from build123d import *

# Parameters (mm, degrees)
SM_BASE_FLANGE_1_DEPTH = 40
SKETCH_6_R             = 1.7
CUT_EXTRUDE_1_DEPTH    = 10
SKETCH_7_R             = 1.7
CUT_EXTRUDE_2_DEPTH    = 10
SKETCH_11_W            = 25.332346726
SKETCH_11_H            = 8.454216192
CUT_EXTRUDE_5_DEPTH    = 10


# Sheet-metal steps are written as plain solids
with BuildPart() as part:
    # Sketch 1 → 基体-法兰1 (new body)
    with BuildSketch(Plane.XY):
        with BuildLine():
            Line((20, 0), (0.5, 0))
            ThreePointArc((0.5, 0), (0.146446609, 0.146446609), (0, 0.5))
            Line((0, 0.5), (0, 15))
            Line((0, 15), (-2, 15))
            Line((-2, 15), (-2, 0.5))
            ThreePointArc((-2, 0.5), (-1.267766953, -1.267766953), (0.5, -2))
            Line((0.5, -2), (20, -2))
            Line((20, -2), (20, 0))
        make_face()
    extrude(amount=SM_BASE_FLANGE_1_DEPTH)

    # 草图6 → 切除-拉伸1 (cut)
    with BuildSketch(Plane(origin=(0, 0, 0), x_dir=(0, 0, -1), z_dir=(1, 0, 0))):
        with Locations((-35, 11)):
            Circle(SKETCH_6_R)
        with Locations((-5, 11)):
            Circle(SKETCH_6_R)
    extrude(amount=-CUT_EXTRUDE_1_DEPTH, mode=Mode.SUBTRACT)

    # 草图7 → 切除-拉伸2 (cut)
    with BuildSketch(Plane(origin=(0, 0, 0), x_dir=(1, 0, 0), z_dir=(0, 1, 0))):
        with Locations(Location((16, -5, 0), (0, 0, 270))):
            Circle(SKETCH_7_R)
        with Locations(Location((16, -35, 0), (0, 0, 270))):
            Circle(SKETCH_7_R)
    extrude(amount=-CUT_EXTRUDE_2_DEPTH, mode=Mode.SUBTRACT)

    # 草图11 → 切除-拉伸5 (cut)
    with BuildSketch(Plane.ZY.offset(2)):
        with Locations((20.136358326, 5.621246346)):
            Rectangle(SKETCH_11_W, SKETCH_11_H)
    extrude(amount=-CUT_EXTRUDE_5_DEPTH, mode=Mode.SUBTRACT)


solid = part.part
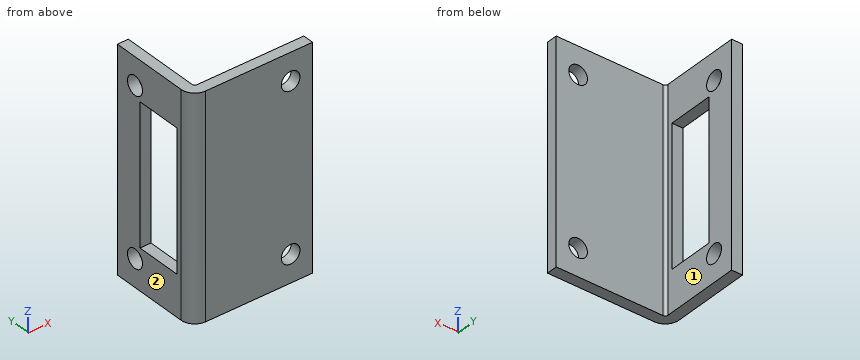
Here's how the part is built. I have some questions about the finished solid (model axes, mm). Face numbers are marked on the shaded views. A direction names the side the tool comes from. Give positions to 0.01 mm unless a question says otherwise; leave off trailing zeros. Loops run counter-clockwise (first coordinate to the right, second up) from the corner with the lowest first, then second, coordinate; pieces in that order, holes last. Notation, with made-up numbers: (33.25, 82) -> (51.25, 82) arc R27 ccw to (51.25, 115) -> close; hole circle Ø7 at (33.25, 81.25). An arc over 180 degrees is marked (long way). One line per item, written item: value.
Q1. Suppose I cut it at A-A on x = 16. Please give me the cut outline in (y, z).
Answers follow:
outline: (-2, 0) -> (0, 0) -> (0, 3.3) -> (-2, 3.3) -> close; (-2, 6.7) -> (0, 6.7) -> (0, 33.3) -> (-2, 33.3) -> close; (-2, 36.7) -> (0, 36.7) -> (0, 40) -> (-2, 40) -> close
Q2. Suppose I cut it at C-C on y = 5.5. Please give me the cut outline in (x, z), then the cut area to 3 significant figures.
Answers follow:
outline: (-2, 0) -> (0, 0) -> (0, 7.47) -> (-2, 7.47) -> close; (-2, 32.8) -> (0, 32.8) -> (0, 40) -> (-2, 40) -> close
area: 29.3 mm^2
Q3. Suppose I cut it at B-B on z = 35. Please give me the cut outline in (x, y).
Answers follow:
outline: (-2, 0.5) arc R2.5 ccw to (0.5, -2) -> (14.3, -2) -> (14.3, 0) -> (0.5, 0) arc R0.5 cw to (0, 0.5) -> (0, 9.3) -> (-2, 9.3) -> close; (-2, 12.7) -> (0, 12.7) -> (0, 15) -> (-2, 15) -> close; (17.7, -2) -> (20, -2) -> (20, 0) -> (17.7, 0) -> close
Q4. Suppose I cut it at D-D on z = 8.5. Please give me the cut outline in (x, y).
Answers follow:
outline: (-2, 0.5) arc R2.5 ccw to (0.5, -2) -> (20, -2) -> (20, 0) -> (0.5, 0) arc R0.5 cw to (0, 0.5) -> (0, 1.39) -> (-2, 1.39) -> close; (-2, 9.85) -> (0, 9.85) -> (0, 15) -> (-2, 15) -> close
Q5. If I drill on line 1 along X through (y, z) = (1.5, 2); line 2 along X through (y, z) = (-1.15, 5), over which ranges is the centre line in solid material (lowest first)?
Answers follow:
line 1: -2 to 0
line 2: -1.38 to 14.3, 17.7 to 20
Q6. I'm going to push flat-ended pins straight in: pin 1 Ø5 at (x, z) = (15.5, 28) entering from +Y; pin 2 Ø10 at (y, z) = (7, 18) entering from +X. Where does each tip first touch, or does it pass through?
Answers follow:
pin 1: y = 0
pin 2: x = 0
Q7. On a 3-axis mill with a long thin cutter (end or side, diameter ignored), from which of +Z, -Z, +X, -X, +Y, -Y can I reach the whole of each face in a straight line? I mean the marked faces 1 and 2. Say none if no direction works.
Answers follow:
face 1: +Z, -Z, +X, +Y
face 2: +Z, -Z, -X, +Y, -Y
